Autodesk Inventor part; units mm, degrees
ref_plane "YZ Plane" through (0, 0, 0) normal (1, 0, 0) x (0, 1, 0)
ref_plane "XZ Plane" through (0, 0, 0) normal (0, 1, 0) x (-1, 0, 0)
ref_plane "XY Plane" through (0, 0, 0) normal (0, 0, 1) x (1, 0, 0)
sketch "Sketch1" plane through (0, 0, 0) normal (0, 0, 1) x (1, 0, 0)
  line L0 (0, 0) -> (50, 0)
  line L1 (50, 0) -> (50, 80) construction
  line L2 (50, 80) -> (0, 80)
  line L3 (0, 80) -> (0, 0)
  circle A0 centre (50, 40) radius 40 construction
  arc A1 (50, 0) -> (50, 80) centre (50, 40) ccw
  dimension "d0" = 50
  dimension "d1" = 80
  dimension "d2" = 80
extrude "Extrusion1" add sketch "Sketch1" along normal blind 40
sketch "Sketch2" plane through (0, 0, 40) normal (0, 0, 1) x (1, 0, 0)
  line L0 (50, 80) -> (0, 80)
  arc A0 (50, 0) -> (50, 80) centre (50, 40) ccw
  line L1 (0, 0) -> (50, 0)
  line L2 (0, 75) -> (50, 75)
  arc A1 (50, 5) -> (50, 75) centre (50, 40) ccw
  line L3 (50, 5) -> (0, 5)
  line L4 (0, 75) -> (0, 5)
  line L5 (0, 80) -> (0, 0)
  dimension "d5" = 5
extrude "Extrusion2" cut sketch "Sketch2" against normal blind 35 contours L2 A1 L3 L4
sketch "Sketch3" plane through (0, 0, 0) normal (-1, 0, 0) x (0, 0, 1)
  line L0 (0, 80) -> (0, 0)
  line L1 (40, 75) -> (40, 5)
  line L2 (0, 80) -> (40, 80)
  line L3 (40, 80) -> (40, 70)
  line L4 (40, 70) -> (0, 70)
  line L5 (0, 70) -> (0, 80)
  line L6 (0, 80) -> (10, 80)
  line L7 (10, 80) -> (10, 50)
  line L8 (10, 50) -> (0, 50)
  line L9 (0, 50) -> (0, 80)
  line L10 (0, 0) -> (40, 0)
  dimension "d8" = 10
  dimension "d9" = 10
  dimension "d10" = 50
extrude "Extrusion3" add sketch "Sketch3" against normal blind 5
sketch "Sketch4" plane through (0, 0, 40) normal (0, 0, 1) x (1, 0, 0)
  line L0 (50, 80) -> (50, 0)
  arc A0 (50, 0) -> (50, 80) centre (50, 40) ccw
  arc A1 (50, 0) -> (50, 80) centre (50, 40) ccw
  arc A2 (50, 0) -> (50, 80) centre (50, 40) ccw
  line L1 (50, 40) -> (40, 80)
  line L2 (50, 80) -> (0, 80)
  line L3 (40, 80) -> (50, 80)
  line L4 (50, 40) -> (40, 0)
  line L5 (0, 0) -> (50, 0)
  line L6 (40, 0) -> (50, 0)
  dimension "d15" = 10
extrude "Extrusion4" cut sketch "Sketch4" against normal blind 10
sketch "Sketch5" plane through (0, 0, 5) normal (0, 0, 1) x (1, 0, 0)
  circle A0 centre (11.5, 30) radius 10
  circle A1 centre (11.5, 30) radius 4.5
  line L0 (0, 0) -> (40, 0)
  line L1 (0, 5) -> (0, 50)
  dimension "d16" = 20
  dimension "d17" = 9
  dimension "d18" = 30
  dimension "d19" = 11.5
extrude "Extrusion5" add sketch "Sketch5" along normal blind 45
sketch "Sketch6" plane through (0, 0, 5) normal (0, 0, 1) x (1, 0, 0)
  circle A0 centre (50, 40) radius 15
  circle A1 centre (50, 40) radius 4.5
  line L0 (0, 5) -> (0, 50)
  line L1 (0, 0) -> (40, 0)
  dimension "d22" = 30
  dimension "d23" = 9
  dimension "d24" = 50
  dimension "d25" = 40
extrude "Extrusion6" add sketch "Sketch6" along normal blind 25
sketch "Sketch7" plane through (0, 0, 5) normal (0, 0, 1) x (1, 0, 0)
  circle A0 centre (15, 65) radius 10
  circle A1 centre (15, 65) radius 2.5
  line L0 (5, 75) -> (41.25, 75)
  line L1 (5, 70) -> (5, 50)
  point P0 (0, 0)
  dimension "d28" = 20
  dimension "d29" = 5
extrude "Extrusion7" add sketch "Sketch7" along normal blind 35
sketch "Sketch9" plane through (0, 0, 0) normal (0, 0, -1) x (-1, 0, 0)
  arc A0 (-15, 75) -> (-5, 65) centre (-15, 65) ccw
  arc A1 (-5, 65) -> (-15, 75) centre (-15, 65) ccw
  circle A2 centre (-15, 65) radius 2.5
  circle A3 centre (-15, 65) radius 2.5
  circle A4 centre (-15, 65) radius 7.5
  point P0 (0, 0)
  dimension "d34" = 15
extrude "Extrusion9" cut sketch "Sketch9" against normal blind 30 contours A2 | A4
sketch "Sketch10" plane through (0, 0, 0) normal (0, 0, -1) x (-1, 0, 0)
  circle A0 centre (-50, 40) radius 15
  circle A1 centre (-11.5, 30) radius 10
  circle A2 centre (-50, 40) radius 2.5
  circle A3 centre (-11.5, 30) radius 10
  circle A4 centre (-11.5, 30) radius 2.5
  point P0 (0, 0)
  dimension "d37" = 5
  dimension "d38" = 5
extrude "Extrusion10" cut sketch "Sketch10" against normal through all contours A2 | A4
properties part number "FA004" material "ABS Plastic"
Source: CAD feature listing. Evaluate the final solid. Frame: model axes, mm. A direction names the side the tool comes from. Coordinates: 2 decimals unless noted, no trailing zeros. Order: outer loops, then holes, each group sorted by start corner. A loop starts at its lowest first (then second) coordinate and runs counter-clockwise, first axis right, second up. Notation, with made-up numbers: M 69,27.5 L 128,27.5 A9 cw 128,36.5 Z; hole C 58.5,-35.5 d4. An arc over 180 degrees is marked long. Write each question's results on one line, items separated by ' | '. Start each with the question number.
1. Section A-A, the plane y = 30. Return the cut outline in (x, z), then the cut area to 3 significant figures.
2. Draft query along Y for faces 4 (the face through (40.634, 77.465, 35.07)), 5 (the face through (5, 72, 22)), 6 (the face through (89.99, 40.88, 14.79)), 7 (the face through (40.634, 2.535, 35.07)). Return one class per face: +Y half, -Y half, draft (parallel to the pull), parting line (faces both ways), or undercut.
3. Section C-C, the plane z = 45.5. Return the cut outline in (x, y).
4. Section B-B, the plane x = 27. Return the cut outline in (y, z), then the cut area to 3 significant figures.
5. Section D-D, the plane y = 46. Return the cut outline in (x, z), then the cut area to 3 significant figures.
6. Material intervals for L1, parallel to Y at x = 50, z = 1.7; L2, parallel to Y at x = 50, z = 17.5; L3, parallel to X at y = 65, z = 37, sorted ascending.
7. Pin query (flat end, axial travel): pin 1 (5.5 mm diameter, centred on x = 29, y = 2.5, fed in from +Z); pin 2 (1.5 mm diameter, centred on x = 19, z = 31.5, fed in from -Y); pin 3 (2.5 mm diameter, centred on x = 12, y = 31.5, fed in from +Z); pin 4 (5 mm diameter, centred on y = 37.5, z = 13, fed in from -X). Return the tip coordinate at first contact, or that it passes through.
8. Reachability of faces 1 (the face through (25, 5, 23)), 2 (the face through (7, 73, 5)), 3 (the face through (53, 44, 30)) from +Z, -Z, +X, -X, +Y, -Y: full face, straight path, thin tool, end or side. Return the list, or none.
Solution:
1) outline: M 0,0 L 9,0 L 9,5 L 7,5 L 7,50 L 1.5,50 L 1.5,5 L 0,5 Z; M 14,0 L 88.73,0 L 88.73,30 L 83.54,30 L 83.54,5 L 61.18,5 L 61.18,30 L 38.82,30 L 38.82,5 L 21.5,5 L 21.5,50 L 16,50 L 16,5 L 14,5 Z | area: 1,600 mm²
2) face 4: +Y half | face 5: undercut | face 6: parting line | face 7: -Y half
3) outline: C 11.5,30 d20; hole C 11.5,30 d9
4) outline: M 0,0 L 80,0 L 80,40 L 75,40 L 75,5 L 5,5 L 5,40 L 0,40 Z | area: 750 mm²
5) outline: M 0,0 L 89.55,0 L 89.55,30 L 84.48,30 L 84.48,5 L 63.75,5 L 63.75,30 L 36.25,30 L 36.25,5 L 0,5 Z | area: 1,260 mm²
6) L1: 0 to 37.5, 42.5 to 80 | L2: 0 to 5, 25 to 35.5, 44.5 to 55, 75 to 80 | L3: 5 to 12.5, 17.5 to 25
7) pin 1: z = 40 | pin 2: y = 0 | pin 3: z = 5 | pin 4: x = 2.84
8) face 1: +Z, -X | face 2: +Z | face 3: +Z, +X
